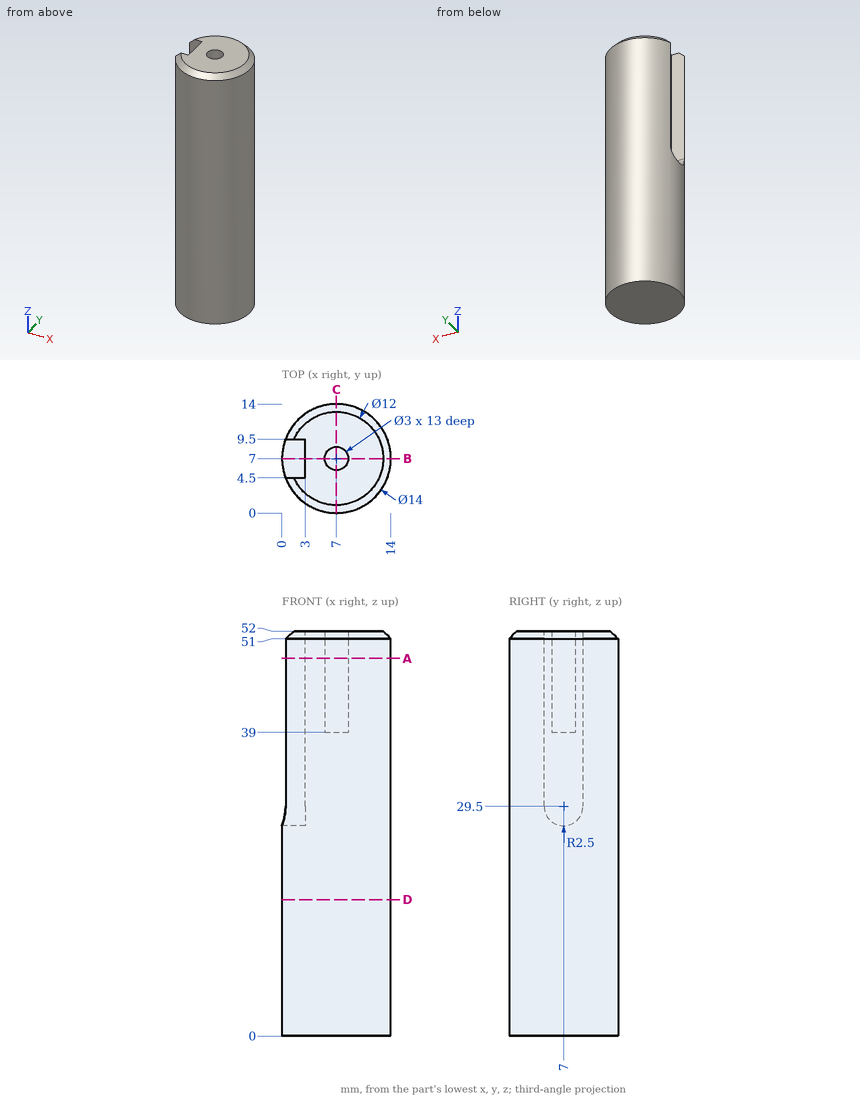
Geometry: see drawing. Coordinates: mm, zero at the bounding-box minimum. Give positions to 0.01 mm unless a question says otherwise; leave off trailing zeros. Loops run counter-clockwise (first coordinate to the right, second up) from the corner with the lowest first, then second, coordinate; pieces in that order, holes last. Notation, with made-up numbers: (-15.5, 61.25) - (28.5, 61.25) arc R11 cw to (28.5, 66.25) - close; hole circle Ø10 at (62.5, 4.5). An arc over 180 degrees is marked (long way). Answer as CSV lines item,"result". Start each with the question number.
1. Pin query (flat end, axial travel): P1, Ø8, axis at x = 2.5, z = 38.5, coming from the -Y side; P2, Ø8, axis at x = 10.5, z = 18.5, coming from the +Y side; P3, Ø0.9, axis at x = 7, y = 7.5, coming from the +Z side; P4, Ø3, axis at y = 12, z = 6.5, coming from the +X side. Return the tip coordinate at first contact, or that it passes through.
2. Ray query, L1, parallel to Y at x = 7.75, z = 46.5; L2, parallel to Y at x = 7.25, z = 11; L3, parallel to Y at x = 9.5, z = 33.5. Return the intervals inside material, ascending.
3. Section C-C, the plane x = 7. Return loops of the section in (y, z).
4. Section B-B, the plane y = 7. Return loops of the section in (x, z), plus the area to 4 significant figures.
5. Section A-A, the plane z = 48.5. Return loops of the section in (x, y), plus the area to 3 significant figures.
6. Section D-D, the plane z = 17.5. Return loops of the section in (x, y), plus the area to 3 significant figures.
Answers:
1,P1,"stops at y = 0.02"
1,P2,"stops at y = 14"
1,P3,"stops at z = 39"
1,P4,"stops at x = 13.06"
2,L1,"y = 0.04 to 5.7, 8.3 to 13.96"
2,L2,"y = 0 to 14"
2,L3,"y = 0.46 to 13.54"
3,outline,"(0, 0) - (14, 0) - (14, 51) - (13, 52) - (8.5, 52) - (8.5, 39) - (5.5, 39) - (5.5, 52) - (1, 52) - (0, 51) - close"
4,outline,"(0, 0) - (14, 0) - (14, 51) - (13, 52) - (8.5, 52) - (8.5, 39) - (5.5, 39) - (5.5, 52) - (3, 52) - (3, 27) - (0, 27) - close"
4,area,"613.5 mm2"
5,outline,"(0.46, 4.5) arc R7 ccw (long way) to (0.46, 9.5) - (3, 9.5) - (3, 4.5) - close; hole circle Ø3 at (7, 7)"
5,area,"133 mm2"
6,outline,"circle Ø14 at (7, 7)"
6,area,"154 mm2"
